```python
from build123d import *

# Parameters (mm, degrees)
SKETCH1_R           = 7
SKETCH1_R_2         = 5
BOSS_EXTRUDE1_DEPTH = 12
CUT_EXTRUDE1_DEPTH  = 40.522145691
FILLET1_R           = 1
BOSS_EXTRUDE2_START = -12
BOSS_EXTRUDE2_DEPTH = 12
FILLET2_R           = 2
CUT_EXTRUDE2_DEPTH  = 59.575636594
SKETCH7_R           = 1
CUT_EXTRUDE3_DEPTH  = 65.110102187


with BuildPart() as part:
    # Sketch1 → Boss-Extrude1 (new body)
    with BuildSketch(Plane(origin=(0, 0, 0), x_dir=(0, 0, -1), z_dir=(1, 0, 0))):
        with Locations((-30, 0)):
            Circle(SKETCH1_R)
        with Locations((-30, 0)):
            Circle(SKETCH1_R_2, mode=Mode.SUBTRACT)
    extrude(amount=BOSS_EXTRUDE1_DEPTH)

    # Sketch3 → Cut-Extrude1 (cut, through all)
    with BuildSketch(Plane(origin=(12, 0, 0), x_dir=(0, 0, -1), z_dir=(1, 0, 0))):
        Polygon((-26, 3), (-26.92060006, -3.93919992), (-40.375880399, -2.154133626), (-39.455280339, 4.785066294), align=None)
    extrude(amount=-CUT_EXTRUDE1_DEPTH, mode=Mode.SUBTRACT)

    # Fillet1
    fillet1_edges = [part.edges().sort_by_distance(p)[0] for p in [
        (6, 3.93919992, 33.07939994),
        (6, 4.266862999, 35.549223383),
        (6, -3, 34),
        (6, -2.672336921, 36.469823443),
    ]]
    fillet(fillet1_edges, radius=FILLET1_R - 0.0001)  # a hair under: the kernel refuses the full size

    # Sketch4 → Boss-Extrude2 (add)
    with BuildSketch(Plane(origin=(12, 0, 0), x_dir=(0, 0, -1), z_dir=(1, 0, 0)).offset(BOSS_EXTRUDE2_START)):
        with BuildLine():
            Line((-23.06080008, -0.92060006), (-16, 40))
            Line((-16, 40), (0, 40))
            Line((0, 40), (0, 45))
            Line((0, 45), (-22, 45))
            Line((-22, 45), (-32.927058907, 6.358641848))
            ThreePointArc((-32.927058907, 6.358641848), (-25.844141537, 5.632835914), (-23.06080008, -0.92060006))
        make_face()
    extrude(amount=BOSS_EXTRUDE2_DEPTH)

    # Fillet2
    fillet2_edges = [part.edges().sort_by_distance(p)[0] for p in [
        (6, 40, 16),
    ]]
    fillet(fillet2_edges, radius=FILLET2_R)

    # Sketch6 → Cut-Extrude2 (cut, through all)
    with BuildSketch(Plane(origin=(12, 0, 0), x_dir=(0, 0, -1), z_dir=(1, 0, 0))):
        with BuildLine():
            Line((-23.744298761, 9.820968741), (-19.349752742, 35.289394134))
            ThreePointArc((-19.349752742, 35.289394134), (-20.381234985, 36.835447129), (-21.979152767, 35.886292641))
            Line((-21.979152767, 35.886292641), (-29.011800399, 11.016740989))
            ThreePointArc((-29.011800399, 11.016740989), (-27.008090108, 7.643460534), (-23.744298761, 9.820968741))
        make_face()
    extrude(amount=-CUT_EXTRUDE2_DEPTH, mode=Mode.SUBTRACT)

    # Mirror9: part across plane


with BuildPart() as part_1:
    add(part.part)
    add(part.part.mirror(Plane(origin=(-56.505687485, 40, 0), x_dir=(1, 0, 0), z_dir=(0, 0, -1))))

    # Sketch7 → Cut-Extrude3 (cut, through all)
    with BuildSketch(Plane(origin=(0, 45, 0), x_dir=(1, 0, 0), z_dir=(0, 1, 0))):
        with Locations(Location((6, -10, 0), (0, 0, 270))):
            Circle(SKETCH7_R)
        with Locations(Location((6, 10, 0), (0, 0, 270))):
            Circle(SKETCH7_R)
    extrude(amount=-CUT_EXTRUDE3_DEPTH, mode=Mode.SUBTRACT)


solid = part_1.part
```
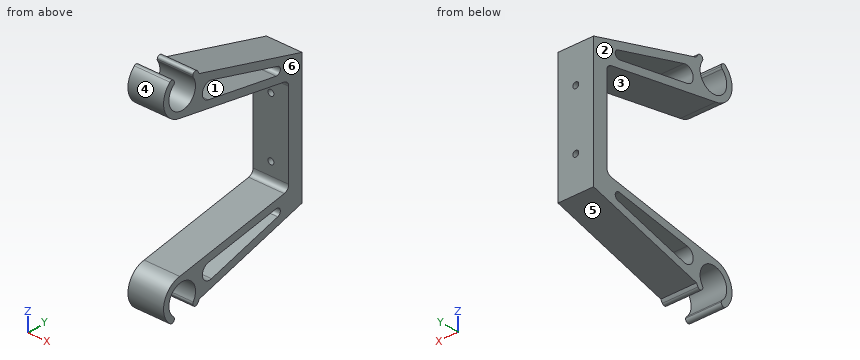
Geometry: final body of the model. Coordinates: model frame, mm. Face numbers are marked on the shaded views. A direction names the side the tool comes from. Give positions to 0.01 mm unless a question says otherwise; leave off trailing zeros. Loops run counter-clockwise (first coordinate to the right, second up) from the corner with the lowest first, then second, coordinate; pieces in that order, holes last. Notation, with made-up numbers: (7.25, 37.25) -> (20.25, 37.25) arc R10 cw to (20.25, 46.25) -> close; hole circle Ø7 at (21, -37). An arc over 180 degrees is marked (long way). Use one line per item in the form item = value.
Item 1: Draft query along Z for the marked faces 4, 5 and 6. Return one class per face: pulls with the +Z half, pulls with the -Z half, needs draft (parallel to the pull), parting line crosses it, or undercut.
A:
face_4 = undercut
face_5 = pulls with the -Z half
face_6 = needs draft
Item 2: Section query A-A on z = -10. Output: boundary loops of the cut face in (x, y).
A:
outline = (0, 40) -> (5, 40) -> (5, 45) -> (0, 45) -> close; (7, 40) -> (12, 40) -> (12, 45) -> (7, 45) -> close
Item 3: Access query for the marked faces 1, 2 and 3. Directions: +Z, -Z, +X, -X, +Y, -Y. A direction counts if a zero-diameter tool reaches every point of the face in a straight line with its end or side. Return the directions, or none.
A:
face_1 = +X, -X
face_2 = +Z, -Z, -X, +Y, -Y
face_3 = +X, -X, -Y
Item 4: Pin query (flat end, axial travel): P1, Ø6, axis at x = 9.5, y = 1.5, coming from the -Z side; P2, Ø4, axis at x = 5.5, y = 21, coming from the -Z side; P3, Ø1.5, axis at x = 5.5, z = 24, coming from the -Y side. Return the tip coordinate at first contact, or that it passes through.
A:
P1 = -34.22
P2 = -29.35
P3 = -4.63
Item 5: Section query C-C on y = 15. Output: boundary loops of the cut face in (x, z).
A:
outline = (0, -30.48) -> (12, -30.48) -> (12, -27.89) -> (0, -27.89) -> close; (0, -22.85) -> (12, -22.85) -> (12, -20.31) -> (0, -20.31) -> close; (0, 20.31) -> (12, 20.31) -> (12, 22.85) -> (0, 22.85) -> close; (0, 27.89) -> (12, 27.89) -> (12, 30.48) -> (0, 30.48) -> close
Item 6: Line query: probe 1 along X at (y, z) = (41, 10); probe 2 along Z at (x, y) = (7.5, 15.5); probe 3 along Z at (x, y) = (11, 13). Output: solid intervals per line, ascending.
A:
probe_1 = 0 to 5, 7 to 12
probe_2 = -30.34 to -27.74, -22.76 to -20.23, 20.23 to 22.76, 27.74 to 30.34
probe_3 = -31.05 to -28.45, -23.2 to -20.66, 20.66 to 23.2, 28.45 to 31.05
Item 7: Section query B-B on x = 1.25. Give the number of separate pieces and of enclosed holes in the cut face, and give its area (3 significant figures).
A:
separate_pieces = 1
enclosed_holes = 2
area = 747 mm^2
Item 8: Section query D-D on y = 0. Output: boundary loops of the cut face in (x, z).
A:
outline = (0, -25) -> (12, -25) -> (12, -22.9) -> (0, -22.9) -> close; (0, 22.9) -> (12, 22.9) -> (12, 25) -> (0, 25) -> close
